from build123d import *

# Parameters (mm, degrees)
SKETCH1_R           = 1.5
SKETCH1_R_2         = 1.25
BOSS_EXTRUDE1_DEPTH = 2


with BuildPart() as part:
    # Sketch1 → Boss-Extrude1 (new body)
    with BuildSketch(Plane(origin=(0, 0, 0), x_dir=(1, 0, 0), z_dir=(0, 1, 0))):
        Polygon((-21.067974578, -3.1615), (-16.567974578, -3.1615), (-16.567974578, 8.7885), (-14.547974578, 9.7685), (4.002025422, 9.8385), (6.022025422, 8.7885), (6.022025422, -3.1615), (10.522025422, -3.1615), (10.522025422, 8.7885), (1.156070136, 13.827789026), (-11.083929864, 13.781600347), (-21.067974578, 8.7885), align=None)
        with Locations(Location((-18.817974578, 2.7885, 0), (0, 0, 270))):
            Circle(SKETCH1_R, mode=Mode.SUBTRACT)
        with Locations(Location((8.272025422, 2.7885, 0), (0, 0, 270))):
            Circle(SKETCH1_R, mode=Mode.SUBTRACT)
        with Locations(Location((-0.723929864, 11.820680446, 0), (0, 0, 270))):
            Circle(SKETCH1_R_2, mode=Mode.SUBTRACT)
    extrude(amount=BOSS_EXTRUDE1_DEPTH)


solid = part.part
The model under review builds one solid part; all positions refer to its coordinate system, in mm. A direction names the side the tool comes from. Coordinates: 2 decimals unless noted, no trailing zeros. Write each loop counter-clockwise with the first axis right and the second up, starting at its lowest first coordinate (ties: lowest second). Pieces come first, ordered by that corner, then holes. Notation, with made-up numbers: (1, 78) - (60, 78) arc R32 ccw to (60, 107) - close; hole circle Ø10 at (-4.5, 48.25). An arc over 180 degrees is marked (long way). Answer as a JSON object with one key per item and string values. Group by question number.
1. Add section C-C (z = -2.25). Give the boundary of the cut face in (x, y).
2. Add section B-B (x = 0). Give the boundary of the cut face in (y, z), plus the area to 3 significant figures.
3. Machinability: for faces 1 (the face through (-15.572, 0.986, -9.272)), 2 (the face through (-1.203, 0.986, -10.666)), which of the approach directions +Z, -Z, +X, -X, +Y, -Y give a long, thin tool a straight path to every point of the face, cutting with its end or side? Answer none if there is none.
4. To check wall thickness, follow probe 1 along X at (y, z) = (0.25, -2.75); probe 2 along X at (y, z) = (0.2, -0.25); probe 3 along X at (y, z) = (0.9, -3.25). State the ranges of each line that lie inside material, in increasing order.
5. Add section A-A (z = -8.25). Give the boundary of the cut face in (x, y), plus the area to 3 significant figures.
6. Mouldability with a two-part tool opening along X and no side actions: class faces 3 (the face through (5.905, 0.986, -11.273)), 4 (the face through (5, 0.99, -9.32)), 5 (the face through (-16.01, 0.99, -11.32)) as pulls with the +X half, pulls with the -X half, needs draft (parallel to the pull), parting line crosses it, or undercut.
7. Add section D-D (y = 0.75). Give the boundary of the cut face in (x, z).
8. Clearance check with a flat-ended pin moving along its axis: pin 1 Ø1.8 at (x, z) = (-18.82, -2.79) entering from -Y. State where the tip first meets the part, or that it passes through.
Findings:
{
 "1": {"outline": "(-21.07, 0) - (-20.22, 0) - (-20.22, 2) - (-21.07, 2) - close; (-17.42, 0) - (-16.57, 0) - (-16.57, 2) - (-17.42, 2) - close; (6.02, 0) - (6.87, 0) - (6.87, 2) - (6.02, 2) - close; (9.67, 0) - (10.52, 0) - (10.52, 2) - (9.67, 2) - close"},
 "2": {"outline": "(0, -13.82) - (2, -13.82) - (2, -12.84) - (0, -12.84) - close; (0, -10.8) - (2, -10.8) - (2, -9.82) - (0, -9.82) - close", "area": "3.92 mm²"},
 "3": {"face 1": "+Z, +Y, -Y", "face 2": "+Y, -Y"},
 "4": {"probe 1": "-21.07 to -20.32, -17.32 to -16.57, 6.02 to 6.77, 9.77 to 10.52", "probe 2": "-21.07 to -16.57, 6.02 to 10.52", "probe 3": "-21.07 to -20.25, -17.39 to -16.57, 6.02 to 6.84, 9.7 to 10.52"},
 "5": {"outline": "(-21.07, 0) - (-16.57, 0) - (-16.57, 2) - (-21.07, 2) - close; (6.02, 0) - (10.52, 0) - (10.52, 2) - (6.02, 2) - close", "area": "18.0 mm²"},
 "6": {"face 3": "pulls with the +X half", "face 4": "undercut", "face 5": "pulls with the -X half"},
 "7": {"outline": "(-21.07, -8.79) - (-11.08, -13.78) - (1.16, -13.83) - (10.52, -8.79) - (10.52, 3.16) - (6.02, 3.16) - (6.02, -8.79) - (4, -9.84) - (-14.55, -9.77) - (-16.57, -8.79) - (-16.57, 3.16) - (-21.07, 3.16) - close; hole circle Ø3 at (-18.82, -2.79); hole circle Ø2.5 at (-0.72, -11.82); hole circle Ø3 at (8.27, -2.79)"},
 "8": {"pin 1": "through"}
}
